Could you check a few things on this model? Use its own coordinates, in mm. Face numbers are marked on the shaded views. A direction names the side the tool comes from. Give positions to 0.01 mm unless a question says otherwise; leave off trailing zeros. Write each loop counter-clockwise with the first axis right and the second up, starting at its lowest first coordinate (ties: lowest second). Pieces come first, ordered by that corner, then holes. Notation, with made-up numbers: (63.25, 47.25) -> (77.25, 47.25) arc R19 cw to (77.25, 51.25) -> close; hole circle Ø7 at (71.25, -27.75). An arc over 180 degrees is marked (long way). One line per question, with ' | ' between items.
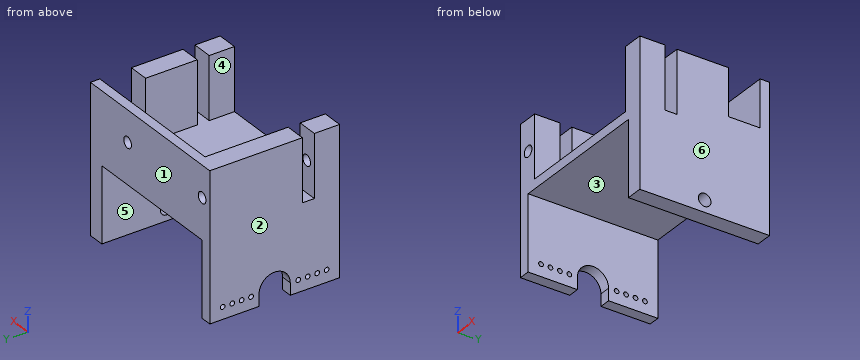
from build123d import *

# Parameters (mm, degrees)
EXTRUDE_1_DEPTH     = 19.8
SKETCH_1_W          = 6.5
SKETCH_1_H          = 8
EXTRUDE_1_2_DEPTH   = 19.8
EXTRUDE_1_3_DEPTH   = 19.8
SKETCH_2_W          = 54.6
SKETCH_2_H          = 41.2
EXTRUDE_2_DEPTH     = 3
SKETCH_4_R          = 0.75
EXTRUDE_3_DEPTH     = 3.5
SKETCH_5_W          = 23.8
SKETCH_5_H          = 41.2
EXTRUDE_4_DEPTH     = 5.2
SKETCH_6_R          = 1.75
CUT_EXTRUDE_2_DEPTH = 8
CUT_EXTRUDE_START   = -8
SKETCH_7_R          = 1.75
CUT_EXTRUDE_3_DEPTH = 8
SKETCH_9_R          = 2
CUT_EXTRUDE_4_DEPTH = 10
SKETCH_10_W         = 14.9
SKETCH_10_H         = 10
CUT_EXTRUDE_5_DEPTH = 7


with BuildPart() as part:
    # Sketch 1 → Extrude 1 (new body)
    with BuildSketch(Plane.XY):
        Polygon((-48.1, 39.2), (-48.1, 12.8), (-54.6, 12.8), (-54.6, 42.2), (-47.6, 42.2), (-7, 42.2), (0, 42.2), (0, 12.8), (-6.5, 12.8), (-6.5, 39.2), align=None)
    extrude(amount=EXTRUDE_1_DEPTH)



with BuildPart() as body_2:
    # Sketch 1 → Extrude 1 2 (new body)
    with BuildSketch(Plane.XY):
        with Locations((-3.25, 5)):
            Rectangle(SKETCH_1_W, SKETCH_1_H)
    extrude(amount=EXTRUDE_1_2_DEPTH)


with BuildPart() as body_3:
    # Sketch 1 → Extrude 1 3 (new body)
    with BuildSketch(Plane.XY):
        with Locations((-51.35, 5)):
            Rectangle(SKETCH_1_W, SKETCH_1_H)
    extrude(amount=EXTRUDE_1_3_DEPTH)


with BuildPart() as part_1:
    add(part.part)

    add(body_2.part)  # Extrude 2 merges body 2

    add(body_3.part)  # Extrude 2 merges body 3
    # Sketch 2 → Extrude 2 (add)
    with BuildSketch(Plane(origin=(0, 0, 0), x_dir=(-1, 0, 0), z_dir=(0, 0, -1))):
        with Locations((27.3, 21.6)):
            Rectangle(SKETCH_2_W, SKETCH_2_H)
    extrude(amount=EXTRUDE_2_DEPTH)

    # Sketch 4 → Extrude 3 (add)
    with BuildSketch(Plane(origin=(-54.6, 54.6, 0), x_dir=(0, -1, 0), z_dir=(1, 0, 0))):
        with BuildLine():
            Line((12.4, 26.8), (28.05, 26.8))
            Line((28.05, 26.8), (28.05, 23))
            ThreePointArc((28.05, 23), (33, 18.05), (37.95, 23))
            Line((37.95, 23), (37.95, 26.8))
            Line((37.95, 26.8), (53.6, 26.8))
            Line((53.6, 26.8), (53.6, 23))
            Line((53.6, 23), (53.6, 3))
            Line((53.6, 3), (12.4, 3))
            Line((12.4, 3), (12.4, 23))
            Line((12.4, 23), (12.4, 26.8))
        make_face()
        with Locations(Location((40.5, 23, 0), (0, 0, 90))):
            Circle(SKETCH_4_R, mode=Mode.SUBTRACT)
        with Locations(Location((43.5, 23, 0), (0, 0, 90))):
            Circle(SKETCH_4_R, mode=Mode.SUBTRACT)
        with Locations(Location((46.5, 23, 0), (0, 0, 90))):
            Circle(SKETCH_4_R, mode=Mode.SUBTRACT)
        with Locations(Location((49.5, 23, 0), (0, 0, 90))):
            Circle(SKETCH_4_R, mode=Mode.SUBTRACT)
        with Locations(Location((16.5, 23, 0), (0, 0, 270))):
            Circle(SKETCH_4_R, mode=Mode.SUBTRACT)
        with Locations(Location((19.5, 23, 0), (0, 0, 270))):
            Circle(SKETCH_4_R, mode=Mode.SUBTRACT)
        with Locations(Location((22.5, 23, 0), (0, 0, 270))):
            Circle(SKETCH_4_R, mode=Mode.SUBTRACT)
        with Locations(Location((25.5, 23, 0), (0, 0, 270))):
            Circle(SKETCH_4_R, mode=Mode.SUBTRACT)
    extrude(amount=EXTRUDE_3_DEPTH)

    # Sketch 5 → Extrude 4 (add)
    with BuildSketch(Plane(origin=(0, 0, 0), x_dir=(0, 0, -1), z_dir=(1, 0, 0))):
        with Locations((14.9, 21.6)):
            Rectangle(SKETCH_5_W, SKETCH_5_H)
    extrude(amount=-EXTRUDE_4_DEPTH)

    # Sketch 6 → Cut-Extrude 2 (cut)
    with BuildSketch(Plane(origin=(0, 1, 0), x_dir=(-1, 0, 0), z_dir=(0, -1, 0))):
        with Locations(Location((51.1, -9.9, 0), (0, 0, 180))):
            Circle(SKETCH_6_R)
    extrude(amount=-CUT_EXTRUDE_2_DEPTH, mode=Mode.SUBTRACT)

    # Sketch 7 → Cut-Extrude 3 (cut)
    with BuildSketch(Plane(origin=(0, 42.2, 0), x_dir=(1, 0, 0), z_dir=(0, 1, 0)).offset(CUT_EXTRUDE_START)):
        with Locations((-51.1, -9.9)):
            Circle(SKETCH_7_R)
        with Locations(Location((-17, -9.9, 0), (0, 0, 270))):
            Circle(SKETCH_7_R)
    extrude(amount=CUT_EXTRUDE_3_DEPTH, mode=Mode.SUBTRACT)

    # Sketch 9 → Cut-Extrude 4 (cut)
    with BuildSketch(Plane(origin=(0, 0, 0), x_dir=(0, 0, -1), z_dir=(1, 0, 0))):
        with Locations(Location((23, 21.6, 0), (0, 0, 90))):
            Circle(SKETCH_9_R)
    extrude(amount=-CUT_EXTRUDE_4_DEPTH, mode=Mode.SUBTRACT)

    # Sketch 10 → Cut-Extrude 5 (cut)
    with BuildSketch(Plane(origin=(0, 0, 0), x_dir=(0, 0, -1), z_dir=(1, 0, 0))):
        with Locations((-12.35, 34.2)):
            Rectangle(SKETCH_10_W, SKETCH_10_H)
    extrude(amount=-CUT_EXTRUDE_5_DEPTH, mode=Mode.SUBTRACT)


solid = part_1.part
Q1. Imagine slicing it at D-D on z = 9.9. Count the separate pieces of the cut face and the enclosed holes in it, and give its area (4 significant figures).
Answer below:
separate pieces: 6 | enclosed holes: 0 | area: 479.5 mm^2
Q2. If we mould it in two halves opening along X, with no side actions, what happens to the marked faces 1, 2 and 3? For each: +X half, -X half, draft (parallel to the pull), parting line (faces both ways), or undercut.
Answer below:
face 1: draft | face 2: -X half | face 3: undercut
Q3. Imagine slicing it at A-A on y = 5.1. Please give me the cut outline in (x, z).
Answer below:
outline: (-54.6, -26.8) -> (-51.1, -26.8) -> (-51.1, -23.75) -> (-54.6, -23.75) -> close; (-54.6, -22.25) -> (-51.1, -22.25) -> (-51.1, -3) -> (-5.2, -3) -> (-5.2, -26.8) -> (0, -26.8) -> (0, 19.8) -> (-6.5, 19.8) -> (-6.5, 0) -> (-48.1, 0) -> (-48.1, 19.8) -> (-54.6, 19.8) -> close; hole circle Ø3.5 at (-51.1, 9.9)
Q4. On a 3-axis mill with a long thin cutter (end or side, diameter ignored), from which of +Z, -Z, +X, -X, +Y, -Y can I reach the whole of each face in a straight line? I mean the marked faces 4, 5 and 6. Say none if no direction works.
Answer below:
face 4: +Z, -Y | face 5: -Z, +Y, -Y | face 6: +Z, -Z, +X, +Y, -Y
Q5. Imagine slicing it at C-C on y = 21.6. Please give me the cut outline in (x, z).
Answer below:
outline: (-54.6, -18.05) -> (-51.1, -18.05) -> (-51.1, -3) -> (-5.2, -3) -> (-5.2, -21) -> (0, -21) -> (0, 19.8) -> (-6.5, 19.8) -> (-6.5, 0) -> (-48.1, 0) -> (-48.1, 19.8) -> (-54.6, 19.8) -> close; (-5.2, -26.8) -> (0, -26.8) -> (0, -25) -> (-5.2, -25) -> close
Q6. Imagine slicing it at B-B on x = -17. Please give me the cut outline in (y, z), and give its area (4 significant figures).
Answer below:
outline: (1, -3) -> (42.2, -3) -> (42.2, 8.15) -> (39.2, 8.15) -> (39.2, 0) -> (1, 0) -> close; (39.2, 11.65) -> (42.2, 11.65) -> (42.2, 19.8) -> (39.2, 19.8) -> close | area: 172.5 mm^2
Q7. If I drill on line 1 along Z through (x, y) = (-52.95, 35.1); line 2 along X through (y, z) = (32, -20.5); line 3 along X through (y, z) = (8, 8.5), over which ranges is the centre line in solid material (lowest first)?
Answer below:
line 1: z = -26.8 to -23.75, -22.25 to 19.8 | line 2: x = -54.6 to -51.1, -5.2 to 0 | line 3: x = -54.6 to -52.15, -50.05 to -48.1, -6.5 to 0
Q8. Will these pins go through, and if not, where does the flat tip stop? pin 1 (2 mm diameter, centred on x = -11, z = 12.5, fed in from -Y); pin 2 (3 mm diameter, centred on x = -51.1, z = 9.9, fed in from +Y); pin 3 (0.9 mm diameter, centred on y = 32.1, z = -23, fed in from -X).
Answer below:
pin 1: stops at y = 39.2 | pin 2: stops at y = 34.2 | pin 3: stops at x = -5.2
